from build123d import *

# Parameters (mm, degrees)
BOSS_EXTRUDE2_START = -8
BOSS_EXTRUDE2_DEPTH = 88
CIRPATTERN1_COUNT   = 8


with BuildPart() as part:
    # Sketch3 → Revolve1 (revolve)
    with BuildSketch(Plane(origin=(0, 0, 0), x_dir=(0, 0, -1), z_dir=(1, 0, 0))):
        Polygon((5, 96), (0, 96), (0, 0), (5, 0), (5, 1), (4.8, 1), (4.8, 2), (5, 2), align=None)
    revolve(axis=Axis((0, 0, 0), (0, 1, 0)))

    # Sketch4 → Boss-Extrude2 (add, through all)
    with BuildSketch(Plane.XZ.offset(BOSS_EXTRUDE2_START)):
        with BuildLine():
            Line((-1, 5.898979486), (-1, 4.898979486))
            ThreePointArc((-1, 4.898979486), (-0.50254481, 4.974680765), (0, 5))
            Line((0, 5), (0, 5.898979486))
            Line((0, 5.898979486), (-1, 5.898979486))
        make_face()
        with BuildLine():
            Line((0, 5.898979486), (0, 5))
            ThreePointArc((0, 5), (0.50254481, 4.974680765), (1, 4.898979486))
            Line((1, 4.898979486), (1, 5.898979486))
            Line((1, 5.898979486), (0, 5.898979486))
        make_face()
    boss_extrude2 = extrude(amount=-BOSS_EXTRUDE2_DEPTH)

    # CirPattern1: Boss-Extrude2 ×8 about axis
    cirpattern1_axis = Axis((0, 0, 0), (0, 1, 0))
    for i in range(1, CIRPATTERN1_COUNT):
        add(boss_extrude2.rotate(cirpattern1_axis, i * 360 / CIRPATTERN1_COUNT))

    # Mirror1: part across plane


with BuildPart() as part_1:
    add(part.part)
    add(part.part.mirror(Plane(origin=(0, 96, 0), x_dir=(0, 0, 1), z_dir=(0, -1, 0))))


solid = part_1.part
Can you work these out from the model? Positions are in its coordinate system, mm. A direction names the side the tool comes from. Give positions to 0.01 mm unless a question says otherwise; leave off trailing zeros. Use one line per item in the form item = value.
1) Will these pins go through, and if not, where does the flat tip stop? pin 1 (0.6 mm diameter, centred on x = -3.5, z = -4.5, fed in from +Y); pin 2 (0.5 mm diameter, centred on x = -5.5, y = 134.5, fed in from -Z); pin 3 (0.6 mm diameter, centred on x = -4.5, z = -4, fed in from -Y).
Answers:
pin_1 = 184
pin_2 = -1
pin_3 = 8
2) I need wall thicknesses on line 1 along X through (y, z) = (67, -4.25); line 2 along Z through (x, y) = (-4.5, 161.5); line 3 along Z through (x, y) = (1.5, 173). Which ranges of each line are inside material? Lowest first, please.
Answers:
line_1 = -4.09 to -2.84, -2.63 to 2.63, 2.84 to 4.09
line_2 = -3.84 to -3.09, -2.18 to 2.18, 3.09 to 3.84
line_3 = -4.77 to 4.77
3) For faces 1 (the face through (0, 192, 0)), 2 (the face through (4.88, 0.51, 1.08)), 3 (the face through (-4.05, 190.49, -2.58)), 4 (the face through (4.88, 191.49, 1.08)), which set-ups out of +Z, -Z, +X, -X, +Y, -Y let a thin tool reach every point of the face, with its end or its side?
Answers:
face_1 = +Z, -Z, +X, -X, +Y
face_2 = -Y
face_3 = none
face_4 = +Y
